Answer from the drawing. Dimensions are ordinates in mm from the lowest x, y and z of the part. A direction names the side the tool comes from. Give positions to 0.01 mm unless a question says otherwise; leave off trailing zeros. Loops run counter-clockwise (first coordinate to the right, second up) from the corner with the lowest first, then second, coordinate; pieces in that order, holes last. Notation, with made-up numbers: (36.25, 44.5) - (79.25, 44.5) arc R13 ccw to (79.25, 52.5) - close; hole circle Ø2 at (37, 27). An arc over 180 degrees is marked (long way). One line per item, written item: value.
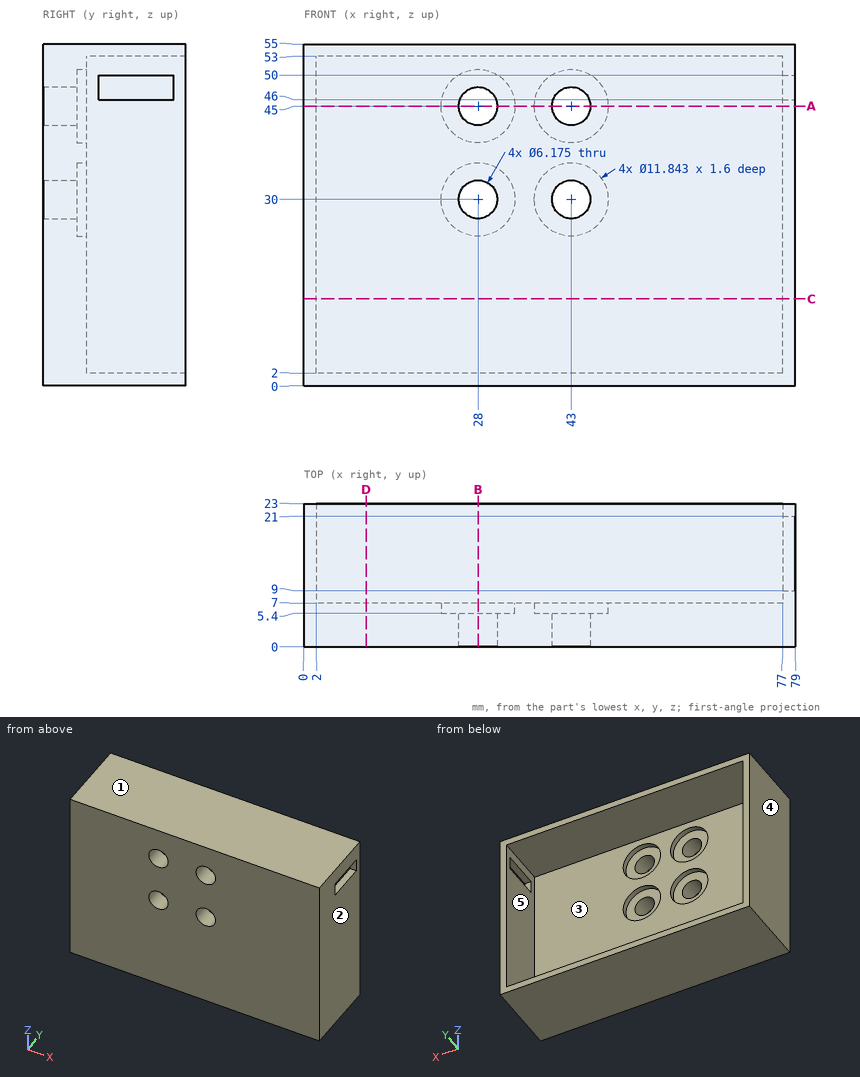
1. Section C-C (z = 14) is taken. Write down the section's boundary in (x, y), and give its area (3 significant figures).
Output:
outline: (0, 0) - (79, 0) - (79, 23) - (77, 23) - (77, 7) - (2, 7) - (2, 23) - (0, 23) - close
area: 617 mm²
2. Section B-B (x = 28) is taken. Write down the section's boundary in (y, z).
Output:
outline: (0, 0) - (23, 0) - (23, 2) - (7, 2) - (7, 24.08) - (5.4, 24.08) - (5.4, 26.91) - (0, 26.91) - close; (0, 33.09) - (5.4, 33.09) - (5.4, 35.92) - (7, 35.92) - (7, 39.08) - (5.4, 39.08) - (5.4, 41.91) - (0, 41.91) - close; (0, 48.09) - (5.4, 48.09) - (5.4, 50.92) - (7, 50.92) - (7, 53) - (23, 53) - (23, 55) - (0, 55) - close
3. Find the intervals of material crossed by line 1 along Z through (x, y) = (28, 5.75); line 2 along X through (y, z) = (3.4, 45); line 3 along Z through (x, y) = (43, 2.9), in increasing order.
Output:
line 1: z = 0 to 24.08, 35.92 to 39.08, 50.92 to 55
line 2: x = 0 to 24.91, 31.09 to 39.91, 46.09 to 79
line 3: z = 0 to 26.91, 33.09 to 41.91, 48.09 to 55
4. Section D-D (x = 10) is taken. Write down the section's boundary in (y, z), and give its area (3 significant figures).
Output:
outline: (0, 0) - (23, 0) - (23, 2) - (7, 2) - (7, 53) - (23, 53) - (23, 55) - (0, 55) - close
area: 449 mm²
5. For the marked faces 4 and 5, determine the directions among +Z, -Z, +X, -X, +Y, -Y from which every point of the face is accessible in a straight line to the end or side of a thin tool.
Output:
face 4: +Z, -Z, -X, +Y, -Y
face 5: +Y
6. The mould has two halves that part along X. Classify the marked faces 1, 2 and 3: released by +X, released by -X, zero draft, split by the parting line, or undercut.
Output:
face 1: zero draft
face 2: released by +X
face 3: undercut
7. Flat-ended cylindrical pins translate along their axes: pin 1 Ø3 at (x, z) = (10.5, 17) entering from +Y; pin 2 Ø3.5 at (x, z) = (42.5, 47) entering from +Y; pin 3 Ø5.5 at (x, z) = (43, 45) entering from +Y. Find the tip coordinate at first contact, or state that the pin passes through.
Output:
pin 1: stops at y = 7
pin 2: stops at y = 5.4
pin 3: passes through
8. Section A-A (z = 45) is taken. Write down the section's boundary in (x, y), and give its area (3 significant figures).
Output:
outline: (0, 0) - (24.91, 0) - (24.91, 5.4) - (22.08, 5.4) - (22.08, 7) - (2, 7) - (2, 23) - (0, 23) - close; (31.09, 0) - (39.91, 0) - (39.91, 5.4) - (37.08, 5.4) - (37.08, 7) - (33.92, 7) - (33.92, 5.4) - (31.09, 5.4) - close; (46.09, 0) - (79, 0) - (79, 23) - (77, 23) - (77, 7) - (48.92, 7) - (48.92, 5.4) - (46.09, 5.4) - close
area: 512 mm²
